Job drawing, mm, ordinate dimensions from the low corner. One solid piece. Round coordinates to 2 decimals unless told otherwise and drop trailing zeros. Write each loop counter-clockwise with the first axis right and the second up, starting at its lowest first coordinate (ties: lowest second). Pieces come first, ordered by that corner, then holes.
1) Drill centre lines: L1, parallel to X at y = 1.3, z = 6.35 (3 decimals); L2, parallel to X at y = 1.7, z = 30.8 (3 decimals). Where is each one in solid material? Low to high.
2) Saw through at A-A on z = 30.8. Write the cut outline in (x, y) (3 decimals), and give its area (3 significant figures).
3) Saw through at C-C on z = 6.35. Write the cut outline in (x, y) (3 decimals).
4) Flat gauge pin, fed straight in: pin 1 (5 mm diameter, centred on x = 19.19, z = 30.8, fed in from +Y). Where does the tip first touch, or does it go through?
5) Saw through at B-B on y = 0.7. Count the separate pieces of the cut face and the enclosed holes in it, and give its area (3 significant figures).
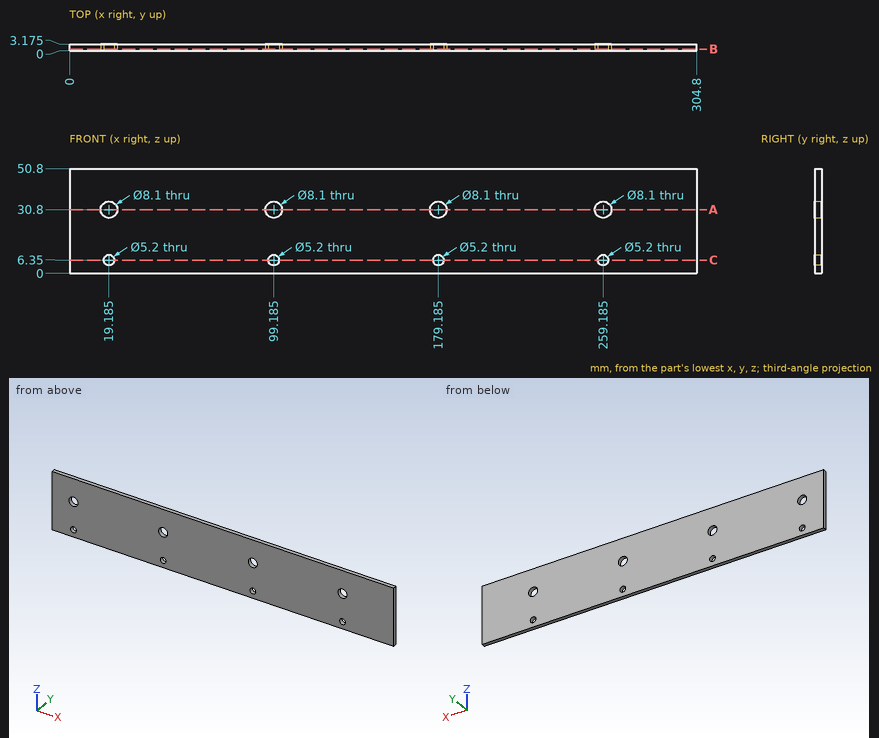
Completed:
1. L1: x = 0 to 16.585, 21.785 to 96.585, 101.785 to 176.585, 181.785 to 256.585, 261.785 to 304.8
1. L2: x = 0 to 15.135, 23.235 to 95.135, 103.235 to 175.135, 183.235 to 255.135, 263.235 to 304.8
2. outline: (0, 0) - (15.135, 0) - (15.135, 3.175) - (0, 3.175) - close; (23.235, 0) - (95.135, 0) - (95.135, 3.175) - (23.235, 3.175) - close; (103.235, 0) - (175.135, 0) - (175.135, 3.175) - (103.235, 3.175) - close; (183.235, 0) - (255.135, 0) - (255.135, 3.175) - (183.235, 3.175) - close; (263.235, 0) - (304.8, 0) - (304.8, 3.175) - (263.235, 3.175) - close
2. area: 865 mm2
3. outline: (0, 0) - (16.585, 0) - (16.585, 3.175) - (0, 3.175) - close; (21.785, 0) - (96.585, 0) - (96.585, 3.175) - (21.785, 3.175) - close; (101.785, 0) - (176.585, 0) - (176.585, 3.175) - (101.785, 3.175) - close; (181.785, 0) - (256.585, 0) - (256.585, 3.175) - (181.785, 3.175) - close; (261.785, 0) - (304.8, 0) - (304.8, 3.175) - (261.785, 3.175) - close
4. pin 1: passes through
5. separate pieces: 1
5. enclosed holes: 8
5. area: 15,200 mm2
